Input: part model. Units: mm. Frame: model coordinates. Face numbers are marked on the shaded views. A direction names the side the tool comes from. Coordinates: 2 decimals unless noted, no trailing zeros. Loops run counter-clockwise (first coordinate to the right, second up) from the corner with the lowest first, then second, coordinate; pieces in that order, holes last.
(1) Section A-A, the plane z = 14.5. Return loops of the section in (x, y) (1 decimal).
(2) Section B-B, the plane y = 30. Return loops of the section in (x, z) (3 decimals).
(3) Section D-D, the plane z = 87. Return loops of the section in (x, y), then the cut area to 3 significant figures.
(4) Mould query, pull axis Y, two halves, no side actions, for the marked faces 1, 2 and 3. Classes: released by +Y, released by -Y, zero draft, split by the parting line, or undercut.
(5) Section C-C, the plane z = 43. Return loops of the section in (x, y), then the cut area to 3 significant figures.
(6) Set-up query: the marked faces 4, 5 and 6. Return all of +Z, -Z, +X, -X, +Y, -Y with unobstructed straight access to the full face (end or side cutting, diameter ignored); none if empty.
(7) Line query: L1, parallel to Z at x = 3, y = 12; L2, parallel to Y at x = -14, z = 52; L3, parallel to Y at x = 16, z = 18. Output: solid intervals per line, ascending.
(8) Contact query for flat-ended pins moving along their axis: P1, Ø3, axis at y = 13.5, z = 25, coming from the -X side; P2, Ø14.5, axis at x = -3, y = -2, coming from the +Z side; P3, Ø6, axis at y = 13.5, z = 57, coming from the +X side; P4, Ø17, axis at y = 26, z = 13, coming from the +X side. Output: stop coordinate, or through.
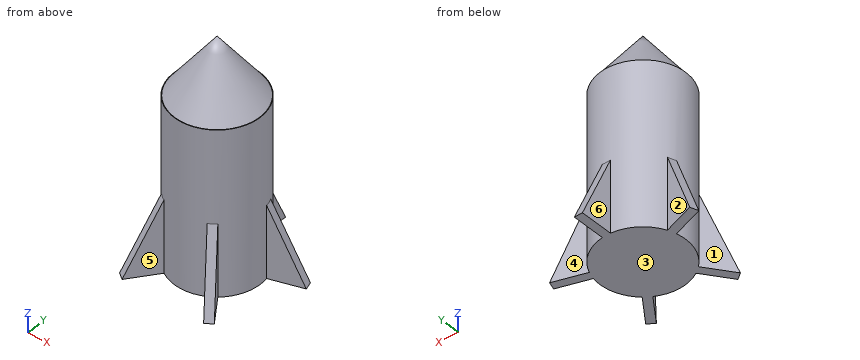
```python
from build123d import *

# Parameters (mm, degrees)
F0_R     = 19.961145
F1_DEPTH = 76.2
F3_DEPTH = 1.905
F4_COUNT = 5


with BuildPart() as f1:
    # F0 (on Top) → F1 (new body)
    with BuildSketch(Plane.XY):
        Circle(F0_R)
    extrude(amount=F1_DEPTH)

    # F2 (on Right) → F3 (join, symmetric)
    with BuildSketch(Plane.YZ):
        Polygon((11.911715, 50.8), (11.911715, 0), (35.1912, 0), align=None)
    extrude(amount=F3_DEPTH, both=True)



with BuildPart() as f4_1:
    # F4: instance of F1
    add(f1.part.rotate(Axis((0, 0, 0), (0, 0, -1)), 1 * 360 / F4_COUNT))


with BuildPart() as f4_2:
    # F4: instance of F1
    add(f1.part.rotate(Axis((0, 0, 0), (0, 0, -1)), 2 * 360 / F4_COUNT))


with BuildPart() as f4_3:
    # F4: instance of F1
    add(f1.part.rotate(Axis((0, 0, 0), (0, 0, -1)), 3 * 360 / F4_COUNT))


with BuildPart() as f4_4:
    # F4: instance of F1
    add(f1.part.rotate(Axis((0, 0, 0), (0, 0, -1)), 4 * 360 / F4_COUNT))


with BuildPart() as f1_1:
    add(f1.part)

    add(f4_1.part)  # F6 merges F4_1

    add(f4_2.part)  # F6 merges F4_2

    add(f4_3.part)  # F6 merges F4_3

    add(f4_4.part)  # F6 merges F4_4
    # F5 (on Right) → F6 (revolve)
    with BuildSketch(Plane.YZ):
        Polygon((-19.869778, 76.00043), (0, 76.300174), (0, 103.126749), align=None)
    revolve(axis=Axis((0, 0, 89.713462), (0, 0, 1)))


solid = f1_1.part
```
Report:
1. outline: (-27.7, 7) - (-19.5, 4.3) arc R20 ccw to (-13.2, -15) - (-18.3, -22) - (-15.2, -24.2) - (-10.1, -17.2) arc R20 ccw to (10.1, -17.2) - (15.2, -24.2) - (18.3, -22) - (13.2, -15) arc R20 ccw to (19.5, 4.3) - (27.7, 7) - (26.6, 10.6) - (18.3, 8) arc R20 ccw to (1.9, 19.9) - (1.9, 28.5) - (-1.9, 28.5) - (-1.9, 19.9) arc R20 ccw to (-18.3, 8) - (-26.6, 10.6) - close
2. outline: (-1.905, 0) - (1.905, 0) - (1.905, 11.328) - (-1.905, 11.328) - close
3. outline: circle Ø23.63 at (0, 0)
3. area: 438 mm2
4. face 1: undercut
4. face 2: released by +Y
4. face 3: zero draft
5. outline: circle Ø39.92 at (0, 0)
5. area: 1,250 mm2
6. face 4: +Z, -Z, +Y
6. face 5: +Z, -Z, -Y
6. face 6: +Z, -Z, -X, +Y
7. L1: z = 0 to 86.24
7. L2: y = -14.23 to 14.23
7. L3: y = -21.68 to -18.78, -11.94 to 11.94
8. P1: stops at x = -15.95
8. P2: stops at z = 103.13
8. P3: stops at x = 16.98
8. P4: stops at x = 9.6
